For this review, take the finished solid that the model builds, in its own axes (mm). A direction names the side the tool comes from. Round coordinates to 2 decimals unless told otherwise and drop trailing zeros. Order: outer loops, then holes, each group sorted by start corner. A loop starts at its lowest first (then second) coordinate and runs counter-clockwise, first axis right, second up. Notation, with made-up numbers: (84, -1.75) -> (130, -1.75) arc R14 ccw to (130, 4.25) -> close; hole circle Ø6 at (-30, -4). An arc over 180 degrees is marked (long way). Answer in a Markdown table with one row per item.
```python
from build123d import *

# Parameters (mm, degrees)
CUT_EXTRUDE1_DEPTH  = 11.78
SKETCH3_W           = 0.4
SKETCH3_H           = 4.6
BOSS_EXTRUDE1_DEPTH = 7.15


with BuildPart() as part:
    # Sketch1 → Revolve1 (revolve)
    with BuildSketch(Plane(origin=(0, 0, 0), x_dir=(0, 0, -1), z_dir=(1, 0, 0)), mode=Mode.PRIVATE) as revolve1_sk:
        Polygon((-2.41, 16.68), (-5.53, 16.68), (-5.53, 11.78), (-3.9, 11.78), (-3.9, 0), (0, 0), (0, 11.78), (-2.41, 11.78), align=None)
    revolve(revolve1_sk.sketch.rotate(Axis((0, 0, 0), (0, 1, 0)), 180), axis=Axis((0, 0, 0), (0, 1, 0)))

    # Sketch2 → Cut-Extrude1 (cut)
    with BuildSketch(Plane.XZ):
        with BuildLine():
            Line((3, -2.491987159), (3, 2.491987159))
            ThreePointArc((3, 2.491987159), (3.9, 0), (3, -2.491987159))
        make_face()
        with BuildLine():
            Line((-3, 2.491987159), (-3, -2.491987159))
            ThreePointArc((-3, -2.491987159), (-3.9, 0), (-3, 2.491987159))
        make_face()
    extrude(amount=-CUT_EXTRUDE1_DEPTH, mode=Mode.SUBTRACT)

    # Sketch3 → Boss-Extrude1 (add)
    with BuildSketch(Plane.XZ):
        Rectangle(SKETCH3_W, SKETCH3_H)
    extrude(amount=BOSS_EXTRUDE1_DEPTH)


solid = part.part
```
Q1. Take a section at A-A, the plane z = 0. Write out the cut boundary in (x, y).
Answer key:
| item | result |
|---|---|
| outline | (-5.53, 11.78) -> (-3, 11.78) -> (-3, 0) -> (-0.2, 0) -> (-0.2, -7.15) -> (0.2, -7.15) -> (0.2, 0) -> (3, 0) -> (3, 11.78) -> (5.53, 11.78) -> (5.53, 16.68) -> (2.41, 16.68) -> (2.41, 11.78) -> (-2.41, 11.78) -> (-2.41, 16.68) -> (-5.53, 16.68) -> close |
Q2. Take a section at B-B, the plane y = 11. Write out the cut boundary in (x, z), then the cut area to 3 significant figures.
Answer key:
| item | result |
|---|---|
| outline | (-3, -2.49) arc R3.9 ccw to (3, -2.49) -> (3, 2.49) arc R3.9 ccw to (-3, 2.49) -> close |
| area | 41.6 mm^2 |
Q3. Clearance check with flat-ended pins moving along their axes: pin 1 Ø5.5 at (y, z) = (4, -0.5) entering from -X; pin 2 Ø4 at (x, y) = (3.5, 2.5) entering from +Z; pin 3 Ø1.5 at (x, y) = (2, 2) entering from -Z. State where each tip first meets the part, or that it passes through.
Answer key:
| item | result |
|---|---|
| pin 1 | stops at x = -3 |
| pin 2 | stops at z = 3.6 |
| pin 3 | stops at z = -3.69 |
Q4. To check wall thickness, follow probe 1 along X at (y, z) = (14.8, 0); probe 2 along Y at (x, z) = (-1.75, -1); probe 3 along Y at (x, z) = (-2.5, -1.25). State the ranges of each line that lie inside material, in increasing order.
Answer key:
| item | result |
|---|---|
| probe 1 | x = -5.53 to -2.41, 2.41 to 5.53 |
| probe 2 | y = 0 to 11.78 |
| probe 3 | y = 0 to 16.68 |
Q5. Tool access review of faces 1 (the face through (0.2, -4, 0)), 2 (the face through (4, 11.78, 0)), 3 (the face through (0, 5.8, -3.9)): name each direction out of +Z, -Z, +X, -X, +Y, -Y from which nothing blocks a thin tool from reaching the whole face with its end or side.
Answer key:
| item | result |
|---|---|
| face 1 | +Z, -Z, +X, -Y |
| face 2 | -Y |
| face 3 | -Z, -Y |
Q6. Take a section at D-D, the plane z = -3.5. Write out the cut boundary in (x, y).
Answer key:
| item | result |
|---|---|
| outline | (-4.28, 11.78) -> (-1.72, 11.78) -> (-1.72, 0) -> (1.72, 0) -> (1.72, 11.78) -> (4.28, 11.78) -> (4.28, 16.68) -> (-4.28, 16.68) -> close |
Q7. The part is to be moulded in two halves that separate along Z. For faces 4 (the face through (0, 5.8, 3.9)), 5 (the face through (3, 6, 0)), 6 (the face through (0, 11.78, 0)), say which applies: +Z half, -Z half, draft (parallel to the pull), parting line (faces both ways), or undercut.
Answer key:
| item | result |
|---|---|
| face 4 | +Z half |
| face 5 | draft |
| face 6 | undercut |
Q8. Take a section at C-C, the plane x = 0.5. Write out the cut boundary in (y, z), then the cut area to 3 significant figures.
Answer key:
| item | result |
|---|---|
| outline | (0, -3.87) -> (11.78, -3.87) -> (11.78, -5.51) -> (16.68, -5.51) -> (16.68, -2.36) -> (11.78, -2.36) -> (11.78, 2.36) -> (16.68, 2.36) -> (16.68, 5.51) -> (11.78, 5.51) -> (11.78, 3.87) -> (0, 3.87) -> close |
| area | 122 mm^2 |
